```python
from build123d import *

# Parameters (mm, degrees)
F0_W     = 673.1
F0_H     = 571.5
F1_DEPTH = 3.175
F2_R     = 2.0701
F3_DEPTH = 25.4
F4_W     = 88.9
F4_H     = 50.8
F5_DEPTH = 25.4


with BuildPart() as f1:
    # F0 (on Front) → F1 (new body)
    with BuildSketch(Plane.XZ):
        Rectangle(F0_W, F0_H)
    extrude(amount=F1_DEPTH)

    # F2 (on face) → F3 (cut)
    with BuildSketch(Plane.XZ.offset(3.175)):
        with Locations((-330.2, -279.4)):
            Circle(F2_R)
        with Locations((-317.5, -279.4)):
            Circle(F2_R)
        with Locations((-317.5, -254)):
            Circle(F2_R)
        with Locations((-330.2, -254)):
            Circle(F2_R)
        with Locations((-330.2, -228.6)):
            Circle(F2_R)
        with Locations((-317.5, -228.6)):
            Circle(F2_R)
        with Locations((-317.5, -203.2)):
            Circle(F2_R)
        with Locations((-330.2, -203.2)):
            Circle(F2_R)
        with Locations((-330.2, -177.8)):
            Circle(F2_R)
        with Locations((-317.5, -177.8)):
            Circle(F2_R)
        with Locations((-317.5, -152.4)):
            Circle(F2_R)
        with Locations((-330.2, -152.4)):
            Circle(F2_R)
        with Locations((-330.2, -127)):
            Circle(F2_R)
        with Locations((-317.5, -127)):
            Circle(F2_R)
        with Locations((-317.5, -101.6)):
            Circle(F2_R)
        with Locations((-330.2, -101.6)):
            Circle(F2_R)
        with Locations((-330.2, -76.2)):
            Circle(F2_R)
        with Locations((-317.5, -76.2)):
            Circle(F2_R)
        with Locations((-317.5, -50.8)):
            Circle(F2_R)
        with Locations((-330.2, -50.8)):
            Circle(F2_R)
        with Locations((-330.2, -25.4)):
            Circle(F2_R)
        with Locations((-317.5, -25.4)):
            Circle(F2_R)
        with Locations((-330.2, 0)):
            Circle(F2_R)
        with Locations((-317.5, 0)):
            Circle(F2_R)
        with Locations((-317.5, 25.4)):
            Circle(F2_R)
        with Locations((-330.2, 25.4)):
            Circle(F2_R)
        with Locations((-330.2, 50.8)):
            Circle(F2_R)
        with Locations((-317.5, 50.8)):
            Circle(F2_R)
        with Locations((-317.5, 76.2)):
            Circle(F2_R)
        with Locations((-330.2, 76.2)):
            Circle(F2_R)
        with Locations((-330.2, 101.6)):
            Circle(F2_R)
        with Locations((-317.5, 101.6)):
            Circle(F2_R)
        with Locations((-330.2, 127)):
            Circle(F2_R)
        with Locations((-317.5, 127)):
            Circle(F2_R)
        with Locations((-317.5, 152.4)):
            Circle(F2_R)
        with Locations((-330.2, 152.4)):
            Circle(F2_R)
        with Locations((-330.2, 177.8)):
            Circle(F2_R)
        with Locations((-317.5, 177.8)):
            Circle(F2_R)
        with Locations((-317.5, 203.2)):
            Circle(F2_R)
        with Locations((-330.2, 203.2)):
            Circle(F2_R)
        with Locations((-330.2, 228.6)):
            Circle(F2_R)
        with Locations((-317.5, 228.6)):
            Circle(F2_R)
        with Locations((-317.5, 254)):
            Circle(F2_R)
        with Locations((-330.2, 254)):
            Circle(F2_R)
        with Locations((-330.2, 279.4)):
            Circle(F2_R)
        with Locations((-317.5, 279.4)):
            Circle(F2_R)
        with Locations((317.5, 279.4)):
            Circle(F2_R)
        with Locations((330.2, 279.4)):
            Circle(F2_R)
        with Locations((317.5, 254)):
            Circle(F2_R)
        with Locations((330.2, 254)):
            Circle(F2_R)
        with Locations((317.5, 228.6)):
            Circle(F2_R)
        with Locations((330.2, 228.6)):
            Circle(F2_R)
        with Locations((317.5, 203.2)):
            Circle(F2_R)
        with Locations((330.2, 203.2)):
            Circle(F2_R)
        with Locations((317.5, 177.8)):
            Circle(F2_R)
        with Locations((330.2, 177.8)):
            Circle(F2_R)
        with Locations((330.2, 152.4)):
            Circle(F2_R)
        with Locations((317.5, 152.4)):
            Circle(F2_R)
        with Locations((317.5, 127)):
            Circle(F2_R)
        with Locations((330.2, 127)):
            Circle(F2_R)
        with Locations((317.5, 101.6)):
            Circle(F2_R)
        with Locations((330.2, 101.6)):
            Circle(F2_R)
        with Locations((330.2, 76.2)):
            Circle(F2_R)
        with Locations((317.5, 76.2)):
            Circle(F2_R)
        with Locations((317.5, 50.8)):
            Circle(F2_R)
        with Locations((330.2, 50.8)):
            Circle(F2_R)
        with Locations((330.2, 25.4)):
            Circle(F2_R)
        with Locations((317.5, 25.4)):
            Circle(F2_R)
        with Locations((317.5, 0)):
            Circle(F2_R)
        with Locations((330.2, 0)):
            Circle(F2_R)
        with Locations((330.2, -25.4)):
            Circle(F2_R)
        with Locations((317.5, -25.4)):
            Circle(F2_R)
        with Locations((317.5, -50.8)):
            Circle(F2_R)
        with Locations((330.2, -50.8)):
            Circle(F2_R)
        with Locations((330.2, -76.2)):
            Circle(F2_R)
        with Locations((317.5, -76.2)):
            Circle(F2_R)
        with Locations((317.5, -101.6)):
            Circle(F2_R)
        with Locations((330.2, -101.6)):
            Circle(F2_R)
        with Locations((317.5, -127)):
            Circle(F2_R)
        with Locations((330.2, -127)):
            Circle(F2_R)
        with Locations((330.2, -152.4)):
            Circle(F2_R)
        with Locations((317.5, -152.4)):
            Circle(F2_R)
        with Locations((317.5, -177.8)):
            Circle(F2_R)
        with Locations((330.2, -177.8)):
            Circle(F2_R)
        with Locations((330.2, -203.2)):
            Circle(F2_R)
        with Locations((317.5, -203.2)):
            Circle(F2_R)
        with Locations((317.5, -228.6)):
            Circle(F2_R)
        with Locations((317.5, -254)):
            Circle(F2_R)
        with Locations((317.5, -279.4)):
            Circle(F2_R)
        with Locations((330.2, -279.4)):
            Circle(F2_R)
        with Locations((330.2, -254)):
            Circle(F2_R)
        with Locations((330.2, -228.6)):
            Circle(F2_R)
    extrude(amount=-F3_DEPTH, mode=Mode.SUBTRACT)

    # F4 (on face) → F5 (cut)
    with BuildSketch(Plane.XZ.offset(3.175)):
        with Locations((-2.54, -248.158)):
            Rectangle(F4_W, F4_H)
        with Locations((-2.54, 248.158)):
            Rectangle(F4_W, F4_H)
    extrude(amount=-F5_DEPTH, mode=Mode.SUBTRACT)


solid = f1.part
```
CAD build for the part. Positions are in the model's coordinates, mm. Round coordinates to 2 decimals unless told otherwise and drop trailing zeros. Return JSON: item names as keys, results as strings. Group by question number.
Item 1: Flat gauge pin, fed straight in: pin 1 Ø3.5 at (x, z) = (-317.5, -25.4) entering from -Y. Where does the tip first touch, or does it go through?
Item 2: Band-saw the part on A-A on y = -0.9. State how many separate pieces and enclosed holes the cut face has, plus the area to 3 significant figures.
Item 3: Probe probe 1 along Z at (x, y) = (-16, -2.75); probe 2 along X at (y, z) = (-1.35, -177.8); probe 3 along X at (y, z) = (-1.2, 254). List the from-to ranges inside material, lowest first.
Item 4: Mould opens along Y. For faces 1 (the face through (-5, 0, 4)), 2 (the face through (-5, -3.175, 4)) say: +Y half, -Y half, draft (parallel to the pull), parting line (faces both ways), or undercut.
Resolved:
{
 "1": {"pin 1": "passes through"},
 "2": {"separate pieces": "1", "enclosed holes": "94", "area": "374,000 mm²"},
 "3": {"probe 1": "z = -285.75 to -273.56, -222.76 to 222.76, 273.56 to 285.75", "probe 2": "x = -336.55 to -332.27, -328.13 to -319.57, -315.43 to 315.43, 319.57 to 328.13, 332.27 to 336.55", "probe 3": "x = -336.55 to -332.27, -328.13 to -319.57, -315.43 to -46.99, 41.91 to 315.43, 319.57 to 328.13, 332.27 to 336.55"},
 "4": {"face 1": "+Y half", "face 2": "-Y half"}
}
